Build history of the part. All positions in model axes, mm. Face numbers are marked on the shaded views. A direction names the side the tool comes from. Round coordinates to 2 decimals unless told otherwise and drop trailing zeros. Write each loop counter-clockwise with the first axis right and the second up, starting at its lowest first coordinate (ties: lowest second). Pieces come first, ordered by that corner, then holes.
Item 1: Drop flat-ended pins along their axis: pin 1 Ø2 at (x, y) = (4, 15) entering from -Z; pin 2 Ø4 at (x, y) = (-280.99, 0) entering from +Z; pin 3 Ø10 at (y, z) = (-14, -13) entering from -X; pin 4 Ø1 at (x, z) = (-151.5, -12) entering from +Y. Give the stop position or say it passes through.
Item 2: Band-saw the part on B-B, the plane x = -37.5. Write the cut outline in (y, z) (1 decimal), then the cut area to 3 significant figures.
Item 3: 3-axis set-ups, long thin cutter, end or side, ignore diameter. For the marked faces 1 and 2: which of +Z, -Z, +X, -X, +Y, -Y reach the whole face in a straight line?
Item 4: Band-saw the part on C-C, the plane y = 12. Write the cut outline in (x, z).
Item 5: Wall check: probe 1 along X at (y, z) = (0, 0.5); probe 2 along X at (y, z) = (15, -4.5); probe 3 along X at (y, z) = (28, -0.5). Give the ranges that are in metal, low to high.
Item 6: Band-saw the part on D-D, the plane z = 28.5. Write the cut outline in (x, y).
```python
from build123d import *

# Parameters (mm, degrees)
F0_R     = 20.6375
F0_R_2   = 6
F1_DEPTH = 268.2875
F2_DEPTH = 287.3375
F3_R     = 3.175
F4_DEPTH = 6.35
F5_START = 239.7125
F0_R_3   = 44.45
F5_DEPTH = 28.575


with BuildPart() as f1:
    # F0 (on Right) → F1 (new body, symmetric)
    with BuildSketch(Plane.YZ):
        Circle(F0_R)
        Circle(F0_R_2, mode=Mode.SUBTRACT)
    extrude(amount=F1_DEPTH, both=True)

    # F0 (on Right) → F2 (join, symmetric)
    with BuildSketch(Plane.YZ):
        Circle(F0_R_2)
    extrude(amount=F2_DEPTH, both=True)

    # F3 (on Top) → F4 (cut, symmetric)
    with BuildSketch(Plane.XY):
        with Locations((-280.9875, 0)):
            Circle(F3_R)
    extrude(amount=F4_DEPTH, both=True, mode=Mode.SUBTRACT)

    # F0 (on Right) → F5 (join)
    with BuildSketch(Plane.YZ.offset(F5_START)):
        Circle(F0_R_3)
        Circle(F0_R, mode=Mode.SUBTRACT)
    extrude(amount=F5_DEPTH)


solid = f1.part
```
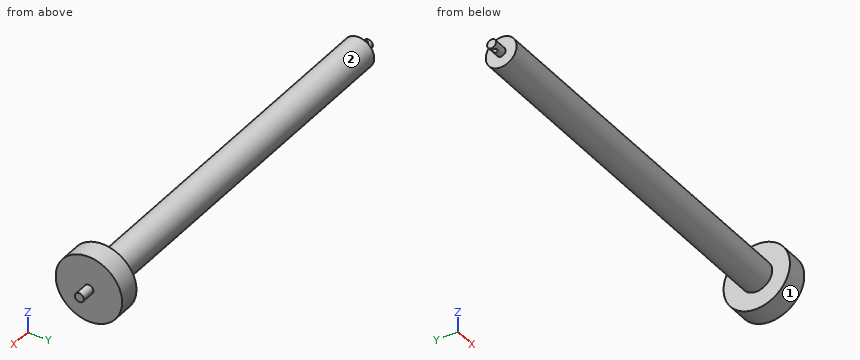
Results:
1. pin 1: stops at z = -15.16
1. pin 2: passes through
1. pin 3: stops at x = -268.29
1. pin 4: stops at y = 17.14
2. outline: circle Ø41.3 at (0, 0)
2. area: 1,340 mm2
3. face 1: +X, -X
3. face 2: -X
4. outline: (-268.29, -16.79) - (239.71, -16.79) - (239.71, -42.8) - (268.29, -42.8) - (268.29, 42.8) - (239.71, 42.8) - (239.71, 16.79) - (-268.29, 16.79) - close
5. probe 1: x = -287.34 to -284.16, -277.81 to 287.34
5. probe 2: x = -268.29 to 268.29
5. probe 3: x = 239.71 to 268.29
6. outline: (239.71, -34.11) - (268.29, -34.11) - (268.29, 34.11) - (239.71, 34.11) - close
